For this review, use the dimensioned drawing (mm, ordinates from the lowest corner) and the shaded views. Coordinates: 2 decimals unless noted, no trailing zeros. Write each loop counter-clockwise with the first axis right and the second up, starting at its lowest first coordinate (ties: lowest second). Pieces come first, ordered by that corner, then holes. Notation, with made-up numbers: (-3.5, -31) - (30.5, -31) arc R31 cw to (30.5, 8) - close; hole circle Ø1 at (-4.5, -20). An arc over 180 degrees is marked (long way). One line per item, written item: value.
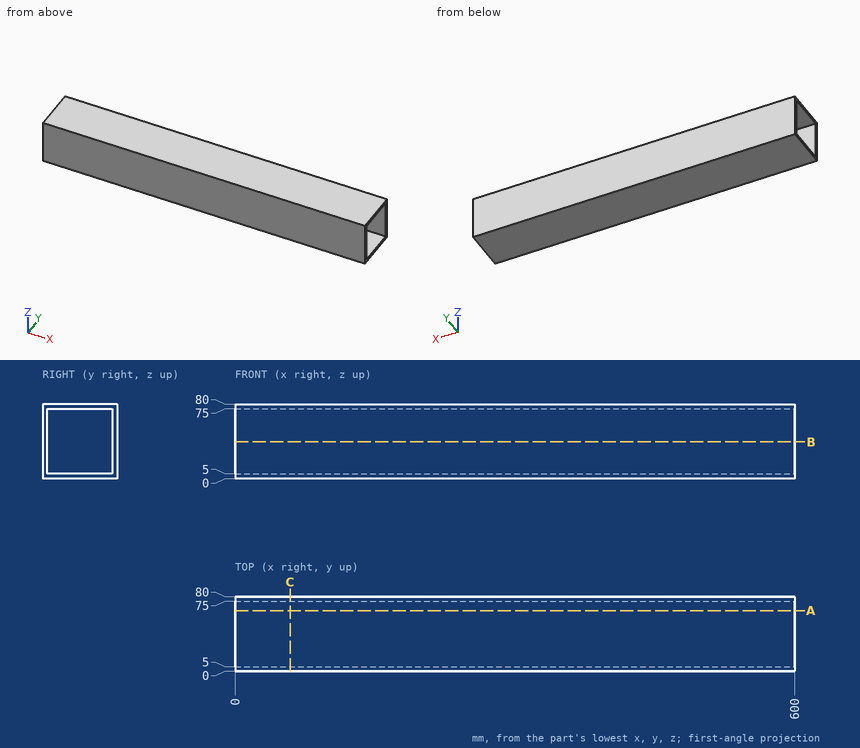
1. Wall thickness on line 1 along Y through (x, z) = (165, 69): over which ranges is the line inside the solid? List them lowest first.
Answer block:
line 1: y = 0 to 5, 75 to 80
2. Consider section C-C, the plane x = 59. Write out the cut boundary in (y, z).
Answer block:
outline: (0, 0) - (80, 0) - (80, 80) - (0, 80) - close; hole (5, 5) - (75, 5) - (75, 75) - (5, 75) - close
3. Consider section A-A, the plane y = 65. Write out the cut boundary in (x, z).
Answer block:
outline: (0, 0) - (600, 0) - (600, 5) - (0, 5) - close; (0, 75) - (600, 75) - (600, 80) - (0, 80) - close
